The model under review builds one solid part; all positions refer to its coordinate system, in mm. Coordinates: 2 decimals unless noted, no trailing zeros. Write each loop counter-clockwise with the first axis right and the second up, starting at its lowest first coordinate (ties: lowest second). Pieces come first, ordered by that corner, then holes. Notation, with made-up numbers: M 78,7 L 127,7 A22 cw 127,46 Z; hole C 38,-7 d1. An arc over 180 degrees is marked long. Answer as a JSON object with one key per item and string values.
```python
from build123d import *

# Parameters (mm, degrees)
SKETCH1_W                 = 254
SKETCH1_H                 = 431.8
BOSS_EXTRUDE1_DEPTH       = 4.3434
SKETCH2_W                 = 8.6868
SKETCH2_H                 = 19.05
SKETCH2_W_2               = 19.05
SKETCH2_H_2               = 8.6868
BOSS_EXTRUDE2_DEPTH       = 4.3434
MIRROR2_COPY_1_SKETCH_W   = 8.6868
MIRROR2_COPY_1_SKETCH_H   = 19.05
MIRROR2_COPY_1_SKETCH_W_2 = 19.05
MIRROR2_COPY_1_SKETCH_H_2 = 8.6868
MIRROR2_COPY_1_DEPTH      = 4.3434


with BuildPart() as part:
    # Sketch1 → Boss-Extrude1 (new body)
    with BuildSketch(Plane.XY):
        Rectangle(SKETCH1_W, SKETCH1_H)
    extrude(amount=BOSS_EXTRUDE1_DEPTH)

    # Sketch2 → Boss-Extrude2 (add)
    with BuildSketch(Plane.XY.offset(4.3434)):
        with Locations((-127, 190.5)):
            Rectangle(SKETCH2_W, SKETCH2_H)
        with Locations((-101.6, 215.9)):
            Rectangle(SKETCH2_W_2, SKETCH2_H_2)
        with Locations((-50.8, 215.9)):
            Rectangle(SKETCH2_W_2, SKETCH2_H_2)
        with Locations((0, 215.9)):
            Rectangle(SKETCH2_W_2, SKETCH2_H_2)
        with Locations((50.8, 215.9)):
            Rectangle(SKETCH2_W_2, SKETCH2_H_2)
        with Locations((101.6, 215.9)):
            Rectangle(SKETCH2_W_2, SKETCH2_H_2)
        with Locations((-127, 136.398)):
            Rectangle(SKETCH2_W, SKETCH2_H)
        with Locations((-127, 82.296)):
            Rectangle(SKETCH2_W, SKETCH2_H)
        with Locations((-127, 28.194)):
            Rectangle(SKETCH2_W, SKETCH2_H)
    boss_extrude2 = extrude(amount=-BOSS_EXTRUDE2_DEPTH)

    # Mirror1: Boss-Extrude2 across plane
    add(boss_extrude2.mirror(Plane(origin=(0, 0, 0), x_dir=(0, 0, 1), z_dir=(1, 0, 0))))

    # Mirror2: Boss-Extrude2 across plane
    add(boss_extrude2.mirror(Plane.ZX))

    # Mirror2 copy 1 sketch → Mirror2 copy 1 (add)
    with BuildSketch(Plane(origin=(0, 0, 4.3434), x_dir=(-1, 0, 0), z_dir=(0, 0, 1))):
        with Locations((-127, 190.5)):
            Rectangle(MIRROR2_COPY_1_SKETCH_W, MIRROR2_COPY_1_SKETCH_H)
        with Locations((-101.6, 215.9)):
            Rectangle(MIRROR2_COPY_1_SKETCH_W_2, MIRROR2_COPY_1_SKETCH_H_2)
        with Locations((-50.8, 215.9)):
            Rectangle(MIRROR2_COPY_1_SKETCH_W_2, MIRROR2_COPY_1_SKETCH_H_2)
        with Locations((0, 215.9)):
            Rectangle(MIRROR2_COPY_1_SKETCH_W_2, MIRROR2_COPY_1_SKETCH_H_2)
        with Locations((50.8, 215.9)):
            Rectangle(MIRROR2_COPY_1_SKETCH_W_2, MIRROR2_COPY_1_SKETCH_H_2)
        with Locations((101.6, 215.9)):
            Rectangle(MIRROR2_COPY_1_SKETCH_W_2, MIRROR2_COPY_1_SKETCH_H_2)
        with Locations((-127, 136.398)):
            Rectangle(MIRROR2_COPY_1_SKETCH_W, MIRROR2_COPY_1_SKETCH_H)
        with Locations((-127, 82.296)):
            Rectangle(MIRROR2_COPY_1_SKETCH_W, MIRROR2_COPY_1_SKETCH_H)
        with Locations((-127, 28.194)):
            Rectangle(MIRROR2_COPY_1_SKETCH_W, MIRROR2_COPY_1_SKETCH_H)
    extrude(amount=-MIRROR2_COPY_1_DEPTH)


solid = part.part
```
(1) Add section B-B on x = 72.5. Give the boundary of the cut face in (y, z).
Results list:
{"outline": "M -215.9,0 L 215.9,0 L 215.9,4.34 L -215.9,4.34 Z"}
(2) Add section A-A on y = 58. Give the boundary of the cut face in (x, z), and give its area (3 significant figures).
Results list:
{"outline": "M -127,0 L 127,0 L 127,4.34 L -127,4.34 Z", "area": "1,100 mm²"}
(3) Wall thickness on line 1 along X through (y, z) = (-177.5, 4.1); line 2 along Y through (x, z) = (89, 1.45): over which ranges is each line inside the solid? List them lowest first. Write a range as from..to.
Results list:
{"line 1": "-127..127", "line 2": "-215.9..215.9"}
(4) For pin 1 Ø1.5 at (y, z) = (-108, 3.5) entering from +X; pin 2 Ø2 at (x, z) = (-129, 3) entering from -Y (3 decimals); pin 3 Ø1.3 at (y, z) = (217, 3) entering from +X (3 decimals), all flat-tipped, find the tip position at first contact; note any pin that passes through.
Results list:
{"pin 1": "x = 127", "pin 2": "y = -200.025", "pin 3": "x = 111.125"}
